Could you check a few things on this drawing? It's one solid part, dimensions in mm from its lowest x, y, z. Coordinates: 2 decimals unless noted, no trailing zeros. Order: outer loops, then holes, each group sorted by start corner. A loop starts at its lowest first (then second) coordinate and runs counter-clockwise, first axis right, second up.
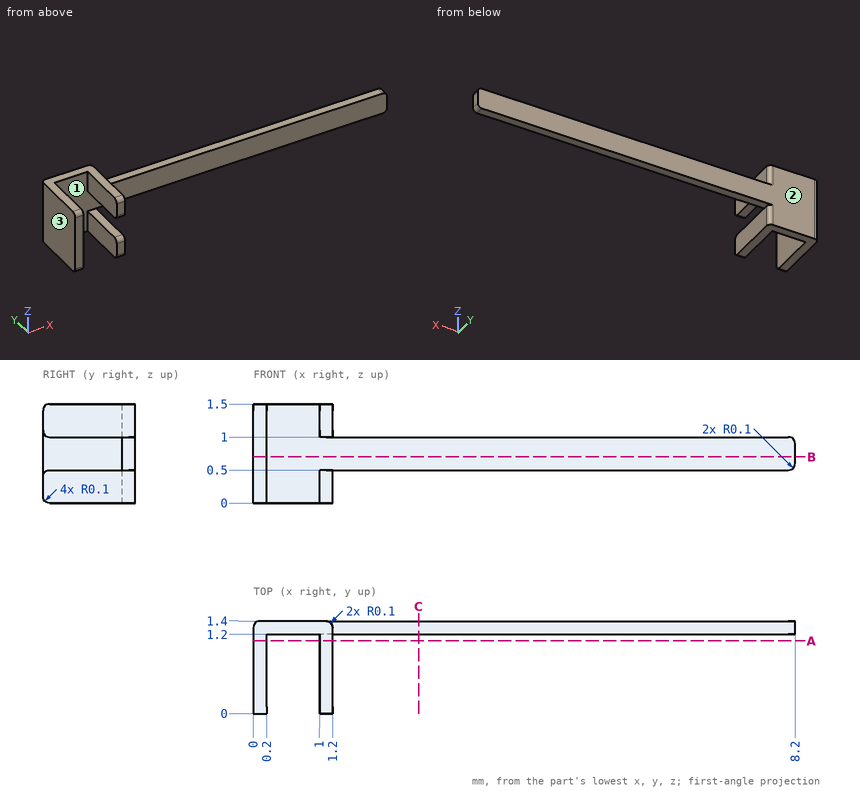
Item 1: Suppose I cut it at B-B (z = 0.7). List the corners of the cut face in (x, y) for me, and give its area (3 significant figures).
Item 2: Thinking about a two-plate mould opening in X: for the marked faces 1, 2 and 3, which applies, +X half, -X half, draft (parallel to the pull), parting line (faces both ways), or undercut?
Item 3: I need wall thicknesses on line 1 (X direction, y = 0.2, z = 0.2); line 2 (Y direction, x = 5, z = 0.65); line 3 (X direction, y = 0.5, z = 0.7). Which ranges of each line are inside material? Lowest first, please.
Item 4: Suppose I cut it at C-C (x = 2.5). List the corners of the cut face in (y, z) for me, and give its area (3 significant figures).
Item 5: Suppose I cut it at A-A (y = 1.1). List the corners of the cut face in (x, z) for me.
Item 6: For pin 1 Ø0.6 at (y, z) = (1, 1) entering from +X, with a flat end and sliding along its axis, tell me the tip position at first contact or that it passes through.
Geometry results:
1. outline: (0, 0) - (0.2, 0) - (0.2, 1.2) - (8.2, 1.2) - (8.2, 1.4) - (0.1, 1.4) arc R0.1 ccw to (0, 1.3) - close
1. area: 1.88 mm2
2. face 1: undercut
2. face 2: draft
2. face 3: -X half
3. line 1: x = 0 to 0.2, 1 to 1.2
3. line 2: y = 1.2 to 1.4
3. line 3: x = 0 to 0.2
4. outline: (1.2, 0.5) - (1.4, 0.5) - (1.4, 1) - (1.2, 1) - close
4. area: 0.100 mm2
5. outline: (0, 0) - (0.2, 0) - (0.2, 1.5) - (0, 1.5) - close; (1, 0) - (1.2, 0) - (1.2, 0.5) - (1, 0.5) - close; (1, 1) - (1.2, 1) - (1.2, 1.5) - (1, 1.5) - close
6. pin 1: stops at x = 8.2
